Source: CAD feature listing. Evaluate the final solid. Frame: model axes, mm. Face numbers are marked on the shaded views. A direction names the side the tool comes from. Round coordinates to 2 decimals unless told otherwise and drop trailing zeros. Write each loop counter-clockwise with the first axis right and the second up, starting at its lowest first coordinate (ties: lowest second). Pieces come first, ordered by that corner, then holes. Notation, with made-up numbers: M 0,66.25 L 5,66.25 A38 ccw 5,105.25 Z; hole C -8,-25.75 d4. An arc over 180 degrees is marked long. Answer in a Markdown table with one row per item.
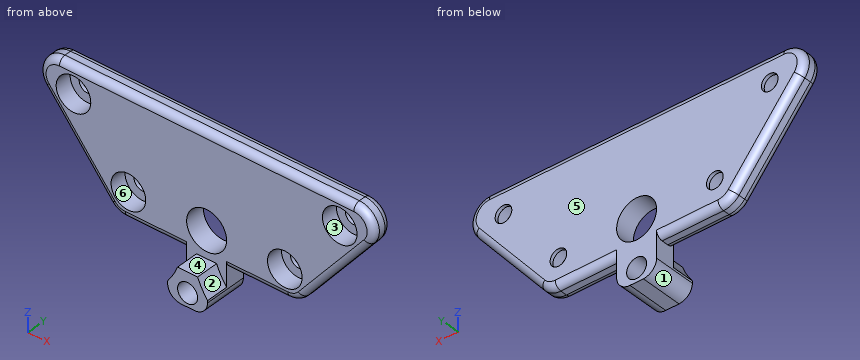
from build123d import *
from build123d.topology import SkipClean

# Parameters (mm, degrees)
SKETCH1_R           = 3
SKETCH1_R_2         = 2.6
SKETCH1_R_3         = 1.5
BOSS_EXTRUDE1_DEPTH = 3
BOSS_EXTRUDE3_START = -0.5
SKETCH3_R           = 2.6
SKETCH3_R_2         = 1.25
BOSS_EXTRUDE3_DEPTH = 0.5
BOSS_EXTRUDE4_START = 3.4
SKETCH4_R           = 1.5
BOSS_EXTRUDE4_DEPTH = 3.4
FILLET1_R           = 1
SKETCH5_R           = 11
CUT_EXTRUDE1_DEPTH  = 3.4


with BuildPart() as part:
    # Sketch1 → Boss-Extrude1 (new body)
    with BuildSketch(Plane(origin=(0, 0, 0), x_dir=(1, 0, 0), z_dir=(0, 1, 0))):
        with BuildLine():
            Line((-14.54167044, 2.903480135), (-24.433461485, -9.146519865))
            ThreePointArc((-24.433461485, -9.146519865), (-24.826727515, -12.332489687), (-22.114676593, -14.05))
            Line((-22.114676593, -14.05), (22.114676593, -14.05))
            ThreePointArc((22.114676593, -14.05), (24.826727515, -12.332489687), (24.433461485, -9.146519865))
            Line((24.433461485, -9.146519865), (14.54167044, 2.903480135))
            ThreePointArc((14.54167044, 2.903480135), (13.505375235, 3.712050922), (12.222885548, 4))
            Line((12.222885548, 4), (3, 4))
            Line((3, 4), (3, 7))
            ThreePointArc((3, 7), (2.414213562, 8.414213562), (1, 9))
            Line((1, 9), (-1, 9))
            ThreePointArc((-1, 9), (-2.414213562, 8.414213562), (-3, 7))
            Line((-3, 7), (-3, 4))
            Line((-3, 4), (-12.222885548, 4))
            ThreePointArc((-12.222885548, 4), (-13.505375235, 3.712050922), (-14.54167044, 2.903480135))
        make_face()
        with Locations(Location((0, 0, 0), (0, 0, 270))):
            Circle(SKETCH1_R, mode=Mode.SUBTRACT)
        with Locations(Location((11.75, 0, 0), (0, 0, 270))):
            Circle(SKETCH1_R_2, mode=Mode.SUBTRACT)
        with Locations(Location((20, -10.05, 0), (0, 0, 270))):
            Circle(SKETCH1_R_2, mode=Mode.SUBTRACT)
        with Locations(Location((-20, -10.05, 0), (0, 0, 90))):
            Circle(SKETCH1_R_2, mode=Mode.SUBTRACT)
        with Locations(Location((-11.75, 0, 0), (0, 0, 90))):
            Circle(SKETCH1_R_2, mode=Mode.SUBTRACT)
        with Locations(Location((0, 7, 0), (0, 0, 270))):
            Circle(SKETCH1_R_3, mode=Mode.SUBTRACT)
    extrude(amount=BOSS_EXTRUDE1_DEPTH)

    # Sketch3 → Boss-Extrude3 (add)
    # profile 1 of 4: a face of its own
    with BuildSketch(Plane(origin=(0, 3, 0), x_dir=(1, 0, 0), z_dir=(0, 1, 0)).offset(BOSS_EXTRUDE3_START)):
        with Locations(Location((-11.75, 0, 0), (0, 0, 90))):
            Circle(SKETCH3_R)
        with Locations(Location((-11.75, 0, 0), (0, 0, 270))):
            Circle(SKETCH3_R_2, mode=Mode.SUBTRACT)
    # profile 2 of 4: a face of its own
    with BuildSketch(Plane(origin=(0, 3, 0), x_dir=(1, 0, 0), z_dir=(0, 1, 0)).offset(BOSS_EXTRUDE3_START)):
        with Locations(Location((-20, -10.05, 0), (0, 0, 90))):
            Circle(SKETCH3_R)
        with Locations(Location((-20, -10.05, 0), (0, 0, 270))):
            Circle(SKETCH3_R_2, mode=Mode.SUBTRACT)
    # profile 3 of 4: a face of its own
    with BuildSketch(Plane(origin=(0, 3, 0), x_dir=(1, 0, 0), z_dir=(0, 1, 0)).offset(BOSS_EXTRUDE3_START)):
        with Locations(Location((11.75, 0, 0), (0, 0, 270))):
            Circle(SKETCH3_R)
        with Locations(Location((11.75, 0, 0), (0, 0, 270))):
            Circle(SKETCH3_R_2, mode=Mode.SUBTRACT)
    # profile 4 of 4: a face of its own
    with BuildSketch(Plane(origin=(0, 3, 0), x_dir=(1, 0, 0), z_dir=(0, 1, 0)).offset(BOSS_EXTRUDE3_START)):
        with Locations(Location((20, -10.05, 0), (0, 0, 270))):
            Circle(SKETCH3_R)
        with Locations(Location((20, -10.05, 0), (0, 0, 270))):
            Circle(SKETCH3_R_2, mode=Mode.SUBTRACT)
    extrude(amount=BOSS_EXTRUDE3_DEPTH)

    # Sketch4 → Boss-Extrude4 (add)
    with SkipClean():  # the faces are left unmerged after this step: merging them gives an invalid solid
        with BuildSketch(Plane(origin=(0, 0, 0), x_dir=(-1, 0, 0), z_dir=(0, -1, 0)).offset(BOSS_EXTRUDE4_START)):
            with BuildLine():
                Line((-3, 4), (-3, 7))
                ThreePointArc((-3, 7), (-2.414213562, 8.414213562), (-1, 9))
                Line((-1, 9), (1, 9))
                ThreePointArc((1, 9), (2.414213562, 8.414213562), (3, 7))
                Line((3, 7), (3, 4))
                Line((3, 4), (-3, 4))
            make_face()
            with Locations(Location((0, 7, 0), (0, 0, 90))):
                Circle(SKETCH4_R, mode=Mode.SUBTRACT)
        extrude(amount=-BOSS_EXTRUDE4_DEPTH)

    # Fillet1
    # the kernel refuses this fillet: 1 mm, written as the material it takes off along each edge
    with BuildSketch(Plane(origin=(-22.114676593, 3, 11.05), x_dir=(-0.772928297309301, 0, -0.6344933783882578), z_dir=(0.6344933783882578, 0, -0.772928297309301))) as fillet1_piece_1:
        with BuildLine():
            CenterArc((3 - FILLET1_R, -FILLET1_R), FILLET1_R, 0, 90)
            Line((3, -FILLET1_R), (3, 0))
            Line((3, 0), (3 - FILLET1_R, 0))
        make_face()
    revolve(axis=Axis((-22.114676593, 3, 11.05), (0, 1, 0)), revolution_arc=129.38241941, mode=Mode.SUBTRACT)
    with BuildSketch(Plane(origin=(-3, 0, -4), x_dir=(0, 1, 0), z_dir=(-1, 0, 0)), Plane(origin=(12.222885548, 3, -4), x_dir=(0, 0, 1), z_dir=(-1, 0, 0))) as fillet1_piece_2:
        with BuildLine():
            CenterArc((FILLET1_R, -FILLET1_R), FILLET1_R, 90, 90)
            Line((0, -FILLET1_R), (0, 0))
            Line((0, 0), (FILLET1_R, 0))
        make_face()
    extrude(amount=9.222885548, mode=Mode.SUBTRACT)
    with BuildSketch(Plane(origin=(12.222885548, 0, -4), x_dir=(0, 0, 1), z_dir=(-1, 0, 0)), Plane(origin=(-3, 3, -4), x_dir=(0, -1, 0), z_dir=(-1, 0, 0))) as fillet1_piece_3:
        with BuildLine():
            CenterArc((FILLET1_R, FILLET1_R), FILLET1_R, 180, 90)
            Line((0, FILLET1_R), (0, 0))
            Line((0, 0), (FILLET1_R, 0))
        make_face()
    extrude(amount=9.222885548, mode=Mode.SUBTRACT)
    with BuildSketch(Plane(origin=(12.222885548, 0, -1), x_dir=(0.7729282973093169, 0, -0.6344933783882384), z_dir=(0.6344933783882384, 0, 0.7729282973093169))) as fillet1_piece_4:
        with BuildLine():
            CenterArc((3 - FILLET1_R, FILLET1_R), FILLET1_R, 270, 90)
            Line((3, FILLET1_R), (3, 0))
            Line((3, 0), (3 - FILLET1_R, 0))
        make_face()
    revolve(axis=Axis((12.222885548, 0, -1), (0, 1, 0)), revolution_arc=50.61758059, mode=Mode.SUBTRACT)
    with BuildSketch(Plane(origin=(-22.114676593, 3, 14.05), x_dir=(0, 0, -1), z_dir=(1, 0, 0))) as fillet1_piece_5:
        with BuildLine():
            CenterArc((FILLET1_R, -FILLET1_R), FILLET1_R, 90, 90)
            Line((0, -FILLET1_R), (0, 0))
            Line((0, 0), (FILLET1_R, 0))
        make_face()
    extrude(amount=44.229353186, mode=Mode.SUBTRACT)
    with BuildSketch(Plane(origin=(24.433461485, 0, 9.146519865), x_dir=(-0.7729282973093136, 0, 0.6344933783882426), z_dir=(-0.6344933783882426, 0, -0.7729282973093136)), Plane(origin=(-14.54167044, 3, -2.903480135), x_dir=(0, -1, 0), z_dir=(-0.6344933783882424, 0, 0.7729282973093137))) as fillet1_piece_6:
        with BuildLine():
            CenterArc((FILLET1_R, FILLET1_R), FILLET1_R, 180, 90)
            Line((0, FILLET1_R), (0, 0))
            Line((0, 0), (FILLET1_R, 0))
        make_face()
    extrude(amount=15.590061901, mode=Mode.SUBTRACT)
    with BuildSketch(Plane(origin=(22.114676593, 0, 11.05), x_dir=(0, 0, 1), z_dir=(-1, 0, 0))) as fillet1_piece_7:
        with BuildLine():
            CenterArc((3 - FILLET1_R, FILLET1_R), FILLET1_R, 270, 90)
            Line((3, FILLET1_R), (3, 0))
            Line((3, 0), (3 - FILLET1_R, 0))
        make_face()
    revolve(axis=Axis((22.114676593, 0, 11.05), (0, 1, 0)), revolution_arc=129.38241941, mode=Mode.SUBTRACT)
    with BuildSketch(Plane(origin=(-22.114676593, 0, 14.05), x_dir=(0, 0, -1), z_dir=(1, 0, 0))) as fillet1_piece_8:
        with BuildLine():
            CenterArc((FILLET1_R, FILLET1_R), FILLET1_R, 180, 90)
            Line((0, FILLET1_R), (0, 0))
            Line((0, 0), (FILLET1_R, 0))
        make_face()
    extrude(amount=44.229353186, mode=Mode.SUBTRACT)
    with BuildSketch(Plane(origin=(-22.114676593, 0, 11.05), x_dir=(-0.772928297309301, 0, -0.6344933783882578), z_dir=(0.6344933783882578, 0, -0.772928297309301))) as fillet1_piece_9:
        with BuildLine():
            CenterArc((3 - FILLET1_R, FILLET1_R), FILLET1_R, 270, 90)
            Line((3, FILLET1_R), (3, 0))
            Line((3, 0), (3 - FILLET1_R, 0))
        make_face()
    revolve(axis=Axis((-22.114676593, 0, 11.05), (0, 1, 0)), revolution_arc=129.38241941, mode=Mode.SUBTRACT)
    with BuildSketch(Plane(origin=(-14.54167044, 0, -2.903480135), x_dir=(0, 1, 0), z_dir=(-0.6344933783882424, 0, 0.7729282973093137)), Plane(origin=(24.433461485, 3, 9.146519865), x_dir=(-0.7729282973093136, 0, 0.6344933783882426), z_dir=(-0.6344933783882426, 0, -0.7729282973093136))) as fillet1_piece_10:
        with BuildLine():
            CenterArc((FILLET1_R, -FILLET1_R), FILLET1_R, 90, 90)
            Line((0, -FILLET1_R), (0, 0))
            Line((0, 0), (FILLET1_R, 0))
        make_face()
    extrude(amount=15.590061901, mode=Mode.SUBTRACT)
    with BuildSketch(Plane(origin=(-12.222885548, 0, -1), x_dir=(0, 0, -1), z_dir=(1, 0, 0))) as fillet1_piece_11:
        with BuildLine():
            CenterArc((3 - FILLET1_R, FILLET1_R), FILLET1_R, 270, 90)
            Line((3 - FILLET1_R, 0), (3, 0))
            Line((3, 0), (3, FILLET1_R))
        make_face()
    revolve(axis=Axis((-12.222885548, 0, -1), (0, 1, 0)), revolution_arc=50.61758059, mode=Mode.SUBTRACT)
    with BuildSketch(Plane(origin=(22.114676593, 3, 11.05), x_dir=(0, 0, 1), z_dir=(-1, 0, 0))) as fillet1_piece_12:
        with BuildLine():
            CenterArc((3 - FILLET1_R, -FILLET1_R), FILLET1_R, 0, 90)
            Line((3, -FILLET1_R), (3, 0))
            Line((3, 0), (3 - FILLET1_R, 0))
        make_face()
    revolve(axis=Axis((22.114676593, 3, 11.05), (0, 1, 0)), revolution_arc=129.38241941, mode=Mode.SUBTRACT)
    with BuildSketch(Plane(origin=(12.222885548, 3, -1), x_dir=(0.7729282973093169, 0, -0.6344933783882384), z_dir=(0.6344933783882384, 0, 0.7729282973093169))) as fillet1_piece_13:
        with BuildLine():
            CenterArc((3 - FILLET1_R, -FILLET1_R), FILLET1_R, 0, 90)
            Line((3, -FILLET1_R), (3, 0))
            Line((3, 0), (3 - FILLET1_R, 0))
        make_face()
    revolve(axis=Axis((12.222885548, 3, -1), (0, 1, 0)), revolution_arc=50.61758059, mode=Mode.SUBTRACT)
    with BuildSketch(Plane(origin=(-12.222885548, 3, -1), x_dir=(0, 0, -1), z_dir=(1, 0, 0))) as fillet1_piece_14:
        with BuildLine():
            CenterArc((3 - FILLET1_R, -FILLET1_R), FILLET1_R, 0, 90)
            Line((3 - FILLET1_R, 0), (3, 0))
            Line((3, 0), (3, -FILLET1_R))
        make_face()
    revolve(axis=Axis((-12.222885548, 3, -1), (0, 1, 0)), revolution_arc=50.61758059, mode=Mode.SUBTRACT)

    # Sketch5 → Cut-Extrude1 (cut)
    with BuildSketch(Plane(origin=(0, -3.4, 0), x_dir=(-1, 0, 0), z_dir=(0, -1, 0))):
        with Locations((-11.75, 0)):
            Circle(SKETCH5_R)
        with Locations((11.75, 0)):
            Circle(SKETCH5_R)
    extrude(amount=-CUT_EXTRUDE1_DEPTH, mode=Mode.SUBTRACT)


solid = part.part
Q1. Access query for the marked faces 5 and 6. Directions: +Z, -Z, +X, -X, +Y, -Y. A direction counts if a zero-diameter tool reaches every point of the face in a straight line with its end or side. Return the directions, or none.
Solutions:
| item | result |
|---|---|
| face 5 | +Z, -Z, +X, -X, +Y |
| face 6 | -Y |
Q2. Pull-direction query (X, two-part tool) for the marked faces 1, 2, 3 and 4; classes: pulls with the +X half, pulls with the -X half, needs draft (parallel to the pull), parting line crosses it, or undercut.
Solutions:
| item | result |
|---|---|
| face 1 | pulls with the -X half |
| face 2 | pulls with the +X half |
| face 3 | undercut |
| face 4 | needs draft |
Q3. Contact query for flat-ended pins moving along their axis: pin 1 Ø2 at (y, z) = (1.5, 3.5) entering from +X; pin 2 Ø8 at (x, z) = (13, -1) entering from -Y; pin 3 Ø1.6 at (x, z) = (-21, 10.5) entering from -Y. Output: stop coordinate, or through.
Solutions:
| item | result |
|---|---|
| pin 1 | stops at x = 20.62 |
| pin 2 | stops at y = 0 |
| pin 3 | stops at y = 2.5 |
Q4. Section B-B (x = 0). Return loops of the section in (y, z), and give its area (3 significant figures).
Solutions:
| item | result |
|---|---|
| outline | M -3.4,-9 L 3,-9 L 3,-8.5 L -3.4,-8.5 Z; M -3.4,-5.5 L 3,-5.5 L 3,-3 L 0,-3 L 0,-4 L -3.4,-4 Z; M 0,3 L 3,3 L 3,13.05 A1 ccw 2,14.05 L 1,14.05 A1 ccw 0,13.05 Z |
| area | 48.5 mm2 |
Q5. Section D-D (z = -0.25). State how many separate pieces and enclosed holes the cut face has, and give its area (3 significant figures).
Solutions:
| item | result |
|---|---|
| separate pieces | 4 |
| enclosed holes | 0 |
| area | 52.9 mm2 |
Q6. Section A-A (y = -2.25). Return loops of the section in (x, z).
Solutions:
| item | result |
|---|---|
| outline | M -3,-7 A2 ccw -1,-9 L 1,-9 A2 ccw 3,-7 L 3,-6.67 A11 cw 1.5,-4 L -1.5,-4 A11 cw -3,-6.67 Z; hole C 0,-7 d3 |
Q7. Section C-C (x = -11.75). Return loops of the section in (y, z), and give its area (3 significant figures).
Solutions:
| item | result |
|---|---|
| outline | M 0,-3 A1 ccw 1,-4 L 2,-4 A1 ccw 3,-3 L 3,-1.25 L 2.5,-1.25 L 2.5,-2.6 L 0,-2.6 Z; M 0,2.6 L 2.5,2.6 L 2.5,1.25 L 3,1.25 L 3,13.05 A1 ccw 2,14.05 L 1,14.05 A1 ccw 0,13.05 Z |
| area | 39.0 mm2 |
Q8. Material intervals for probe 1 along Z at (x, y) = (-11.75, 1.1); probe 2 along X at (y, z) = (0.95, 10.05); probe 3 along X at (y, z) = (2.65, 0), sorted ascending.
Solutions:
| item | result |
|---|---|
| probe 1 | z = -4 to -2.6, 2.6 to 14.05 |
| probe 2 | x = -24.94 to -22.6, -17.4 to 17.4, 22.6 to 24.94 |
| probe 3 | x = -16.61 to -13, -10.5 to -3, 3 to 10.5, 13 to 16.61 |
